Geometry check sheet. Reference: the model listing, model coordinates, mm. A direction names the side the tool comes from. Give positions to 0.01 mm unless a question says otherwise; leave off trailing zeros. Order: outer loops, then holes, each group sorted by start corner. A loop starts at its lowest first (then second) coordinate and runs counter-clockwise, first axis right, second up. Notation, with made-up numbers: M 36,52.5 L 83,52.5 A5 cw 83,60.5 Z; hole C 3.25,70.5 d2. An arc over 180 degrees is marked long. Put each result on its own line as item: value. Start each with the question number.
Q1. Section check C-C on z = 0.5. Record the cut outline in (x, y).
Q2. Section check A-A on y = 0. Record the cut outline in (x, z), then the cut area to 4 significant figures.
Q3. Material ranges on L1, parallel to Y at x = 14, z = 1.1; L2, parallel to Z at x = -12, y = 3.75; L3, parallel to Z at x = 6.5, y = 4, recorded low to high.
Q4. Access from +Z, -Z, +X, -X, +Y, -Y to the whole of each face (thin tool, end or side, straight path). Record for faces 1 (the flat face through (5, 0, 0)), 2 (the flat face through (8.5, -0.1, 3.5)), 3 (the flat face through (-16, 0, -3)).
Q5. Section check B-B on x = 14. Record the cut outline in (y, z).
Q6. Mould release check, pull along X, two halves, no side actions. Record for faces 4 (the cylindrical face through (12.4, 0.07, 2.03)), 5 (the flat face through (-6, 0, 3)), 6 (the flat face through (-20, 0, 0)): +X half, -X half, draft (parallel to the pull), parting line (faces both ways), or undercut.
Q7. Go/stop test with flat-tipped pins: pin 1 (1 mm diameter, centred on x = 7.5, y = -0.5, fed in from -Z); pin 2 (1.9 mm diameter, centred on x = 14, y = 0, fed in from -Z); pin 3 (3.5 mm diameter, centred on x = -14, y = 0, fed in from +Z); pin 4 (1.5 mm diameter, centred on y = -2, z = -2, fed in from +X). Record where each tip stops, or that it passes through.
Q8. Section check D-D on z = -2.5. Record the cut outline in (x, y).
```python
from build123d import *

# Parameters (mm, degrees)
SKETCH_1_W               = 35
SKETCH_1_H               = 10
EXTRUDE_1_DEPTH          = 3
SKETCH_2_W               = 9
SKETCH_2_H               = 10
EXTRUDE_2_DEPTH          = 1
SKETCH_3_R               = 1
EXTRUDE_3_DEPTH          = 8
SKETCH_4_W               = 6
SKETCH_4_H               = 10
EXTRUDE_4_DEPTH          = 3
SKETCH_5_R               = 1.5
CUT_EXTRUDE_1_DEPTH      = 6
SKETCH_6_W               = 6
SKETCH_6_H               = 10
EXTRUDE_5_DEPTH          = 5
SKETCH_7_R               = 1.6
CUT_EXTRUDE_2_DEPTH      = 8
CUT_EXTRUDE_2_DEPTH_BACK = 4
SKETCH_8_W               = 4
SKETCH_8_H               = 10
EXTRUDE_6_DEPTH          = 2.5
SKETCH_10_R              = 1.6
CUT_EXTRUDE_3_DEPTH      = 7
SKETCH_11_W              = 3
SKETCH_11_H              = 10
EXTRUDE_7_DEPTH          = 2.5
SKETCH_12_W              = 6
SKETCH_12_H              = 10
CUT_EXTRUDE_4_DEPTH      = 2.5


with BuildPart() as part:
    # 草圖1 → 填料-伸長1 (new body)
    with BuildSketch(Plane.XY):
        Rectangle(SKETCH_1_W, SKETCH_1_H)
    extrude(amount=EXTRUDE_1_DEPTH)

    # 草圖2 → 填料-伸長2 (add)
    with BuildSketch(Plane.XY.offset(3)):
        with Locations((13, 0)):
            Rectangle(SKETCH_2_W, SKETCH_2_H)
    extrude(amount=EXTRUDE_2_DEPTH)

    # 草圖3 → 填料-伸長3 (add)
    with BuildSketch(Plane.XY.offset(4)):
        with Locations((14, 0)):
            Circle(SKETCH_3_R)
    extrude(amount=EXTRUDE_3_DEPTH)

    # 草圖4 → 填料-伸長4 (add)
    with BuildSketch(Plane(origin=(0, 0, 0), x_dir=(-1, 0, 0), z_dir=(0, 0, -1))):
        with Locations((14.5, 0)):
            Rectangle(SKETCH_4_W, SKETCH_4_H)
    extrude(amount=EXTRUDE_4_DEPTH)

    # 草圖5 → 除料-伸長1 (cut)
    with BuildSketch(Plane(origin=(0, 0, -3), x_dir=(-1, 0, 0), z_dir=(0, 0, -1))):
        with Locations((14, 0)):
            Circle(SKETCH_5_R)
    extrude(amount=-CUT_EXTRUDE_1_DEPTH, mode=Mode.SUBTRACT)

    # 草圖6 → 填料-伸長5 (add)
    with BuildSketch(Plane.ZY.offset(17.5)):
        Rectangle(SKETCH_6_W, SKETCH_6_H)
    extrude(amount=EXTRUDE_5_DEPTH)

    # 草圖7 → 除料-伸長2 (cut, two sides)
    with BuildSketch(Plane.XY.offset(4)) as cut_extrude_2_sk:
        with Locations((14, 0)):
            Circle(SKETCH_7_R)
    extrude(amount=CUT_EXTRUDE_2_DEPTH, mode=Mode.SUBTRACT)
    extrude(cut_extrude_2_sk.sketch, amount=-CUT_EXTRUDE_2_DEPTH_BACK, mode=Mode.SUBTRACT)

    # 草圖8 → 填料-伸長6 (add)
    with BuildSketch(Plane(origin=(17.5, 0, 0), x_dir=(0, 0, -1), z_dir=(1, 0, 0))):
        with Locations((-2, 0)):
            Rectangle(SKETCH_8_W, SKETCH_8_H)
    extrude(amount=EXTRUDE_6_DEPTH)

    # 草圖10 → 除料-伸長3 (cut)
    with BuildSketch(Plane(origin=(0, 0, -3), x_dir=(-1, 0, 0), z_dir=(0, 0, -1))):
        with Locations((14, 0)):
            Circle(SKETCH_10_R)
    extrude(amount=-CUT_EXTRUDE_3_DEPTH, mode=Mode.SUBTRACT)

    # 草圖11 → 填料-伸長7 (add)
    with BuildSketch(Plane(origin=(-11.5, 0, 0), x_dir=(0, 0, -1), z_dir=(1, 0, 0))):
        with Locations((1.5, 0)):
            Rectangle(SKETCH_11_W, SKETCH_11_H)
    extrude(amount=EXTRUDE_7_DEPTH)

    # 草圖12 → 除料-伸長4 (cut)
    with BuildSketch(Plane.ZY.offset(22.5)):
        Rectangle(SKETCH_12_W, SKETCH_12_H)
    extrude(amount=-CUT_EXTRUDE_4_DEPTH, mode=Mode.SUBTRACT)


solid = part.part
```
Results found:
1. outline: M -20,-5 L 20,-5 L 20,5 L -20,5 Z; hole C -14,0 d3.2; hole C 14,0 d3.2
2. outline: M -20,-3 L -15.6,-3 L -15.6,3 L -20,3 Z; M -12.4,-3 L -9,-3 L -9,0 L 12.4,0 L 12.4,4 L 8.5,4 L 8.5,3 L -12.4,3 Z; M 15.6,0 L 20,0 L 20,4 L 15.6,4 Z
2. area: 132.5 mm^2
3. L1: y = -5 to -1.6, 1.6 to 5
3. L2: z = -3 to 3
3. L3: z = 0 to 3
4. face 1: -Z, +X, +Y, -Y
4. face 2: +Z, -X, +Y, -Y
4. face 3: -Z, +X, -X, +Y, -Y
5. outline: M -5,0 L -1.6,0 L -1.6,4 L -5,4 Z; M 1.6,0 L 5,0 L 5,4 L 1.6,4 Z
6. face 4: undercut
6. face 5: draft
6. face 6: -X half
7. pin 1: stops at z = 0
7. pin 2: passes through
7. pin 3: stops at z = 3
7. pin 4: stops at x = -9
8. outline: M -20,-5 L -9,-5 L -9,5 L -20,5 Z; hole C -14,0 d3.2
